For this review, use the dimensioned drawing (mm, ordinates from the lowest corner) and the shaded views. Give positions to 0.01 mm unless a question says otherwise; leave off trailing zeros. Write each loop counter-clockwise with the first axis right and the second up, starting at its lowest first coordinate (ties: lowest second). Pieces come first, ordered by that corner, then holes. Notation, with made-up numbers: (1.25, 87.25) -> (37.25, 87.25) arc R25 ccw to (37.25, 107.25) -> close; hole circle Ø2 at (34, 25). An arc over 180 degrees is marked (long way). Answer as CSV lines item,"result".
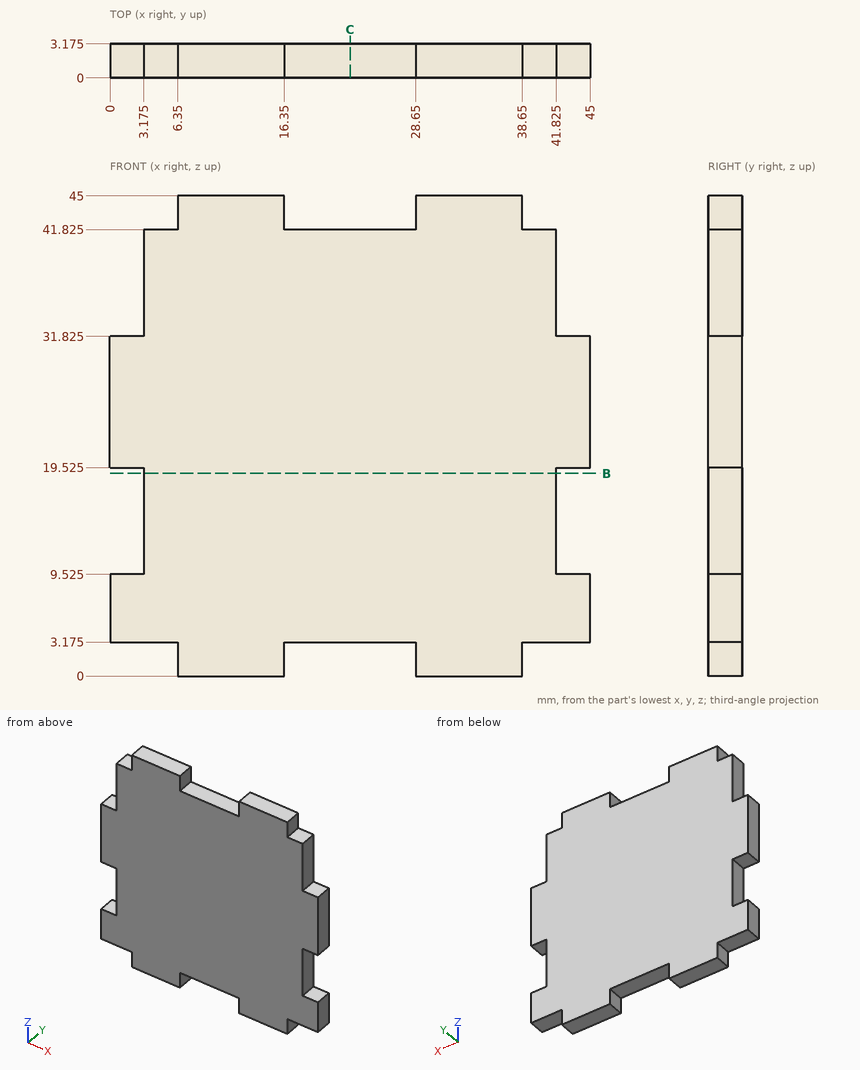
Q1. Add section B-B (z = 19). Write out the cut boundary in (x, y) (3 decimals), plus the area to 3 significant figures.
Answer block:
outline,"(3.175, 0) -> (41.825, 0) -> (41.825, 3.175) -> (3.175, 3.175) -> close"
area,"123 mm2"
Q2. To check wall thickness, follow probe 1 along Z at (x, y) = (43.5, 0.35) (3 decimals); probe 2 along X at (y, z) = (0.45, 15.5) (3 decimals). State the ranges of each line that lie inside material, in increasing order. Write a range as [from, to].
Answer block:
probe 1,"z = [3.175, 9.525], [19.525, 31.825]"
probe 2,"x = [3.175, 41.825]"
Q3. Clearance check with flat-ended pins moving along their axes: pin 1 (1 mm diameter, centred on x = 2, y = 2, fed in from +Z) (3 decimals); pin 2 (1.6 mm diameter, centred on y = 1, z = 43.5, fed in from -X); pin 3 (1.5 mm diameter, centred on x = 20.5, z = 16.5, fed in from -Y); pin 4 (1 mm diameter, centred on x = 4, y = 1.5, fed in from +Z) (3 decimals). State where each tip first meets the part, or that it passes through.
Answer block:
pin 1,"stops at z = 31.825"
pin 2,"stops at x = 6.35"
pin 3,"stops at y = 0"
pin 4,"stops at z = 41.825"
Q4. Add section C-C (x = 22.5). Write out the cut boundary in (y, z) (3 decimals).
Answer block:
outline,"(0, 3.175) -> (3.175, 3.175) -> (3.175, 41.825) -> (0, 41.825) -> close"
